Verification items for the finished model (mm, model axes). A direction names the side the tool comes from. Round coordinates to 2 decimals unless told otherwise and drop trailing zeros. Order: outer loops, then holes, each group sorted by start corner. A loop starts at its lowest first (then second) coordinate and runs counter-clockwise, first axis right, second up. Notation, with made-up numbers: (-11, 28.5) -> (46, 28.5) arc R29 ccw to (46, 63.5) -> close; hole circle Ø8 at (76.25, -10). An arc over 180 degrees is marked (long way). Return JSON: item names as keys, results as strings. Group by question number.
1) Section check B-B on y = -21. Enter the section's corners in (x, z).
2) Section check A-A on x = 363. Enter the section's corners in (y, z), plus the area to 3 significant figures.
3) Depth check by flat-ended pin: pin 1 (8 mm diameter, centred on x = 1498.6, z = -27.305, fed in from -Y); pin 2 (5.5 mm diameter, centred on x = 3.81, z = -33.34, fed in from +Y); pin 3 (8 mm diameter, centred on x = 532.5, y = -24, fed in from -Z); pin 4 (6 mm diameter, centred on y = -29.5, z = -4.5, fed in from -X). Enter the tip coordinate at first touch or a pass-through.
4) Tool access check on faces 1 (the flat face through (742, 0, -28)), 2 (the flat face through (742, -2.591, -28)). Record the directions out of +Z, -Z, +X, -X, +Y, -Y that give a thin tool (end or side, any length) a straight path to the whole face; none if there is none.
5) Scan lines: L1, parallel to Z at x = 1498.6, y = -0.85; L2, parallel to Z at x = 3.81, y = -0.65; L3, parallel to Y at x = 86.5, z = -31. Record each from-to range of solid material in increasing order.
```python
from build123d import *

# Parameters (mm, degrees)
BASE_FLANGE1_DEPTH               = 2.5908
EDGE_FLANGE1_STRIP_W             = 15.4432
EDGE_FLANGE1_STRIP_H             = 2.5908
EDGE_FLANGE1_STRIP_CUT_DEPTH     = 1524
EDGE_FLANGE1_DEPTH               = 1524
F_17_64_0_26563_DIAMETER_HOLE1_D = 6.747002
FILLET1_R                        = 3.175
F_17_64_0_26563_DIAMETER_HOLE2_D = 6.747002


# Sheet-metal steps are written as plain solids
with BuildPart() as part:
    # Sketch2 → Base-Flange1 (new body)
    with BuildSketch(Plane(origin=(0, 0, 0), x_dir=(1, 0, 0), z_dir=(0, 1, 0))):
        Polygon((0, 0), (1524, 0), (1524, 50.8), (-19.05, 50.8), (-19.05, 19.05), (0, 9.525), align=None)
    extrude(amount=-BASE_FLANGE1_DEPTH)

    # Edge-Flange1 strip (across the edge) → Edge-Flange1 strip cut (cut)
    with BuildSketch(Plane(origin=(1524, -2.5908, 0), x_dir=(0, 0, -1), z_dir=(-1, 0, 0))):
        with Locations((-2.5908, -1.2954)):
            Rectangle(EDGE_FLANGE1_STRIP_W, EDGE_FLANGE1_STRIP_H)
    extrude(amount=EDGE_FLANGE1_STRIP_CUT_DEPTH, mode=Mode.SUBTRACT)

    # Edge-Flange1 section (across the edge) → Edge-Flange1 (add)
    with BuildSketch(Plane(origin=(1524, -2.5908, 0), x_dir=(0, 0, -1), z_dir=(-1, 0, 0))):
        with BuildLine():
            Line((0, 2.54), (0, 48.2092))
            Line((0, 48.2092), (2.5908, 48.2092))
            Line((2.5908, 48.2092), (2.5908, 2.54))
            ThreePointArc((2.5908, 2.54), (3.334748776, 0.743948776), (5.1308, 0))
            Line((5.1308, 0), (5.1308, -2.5908))
            ThreePointArc((5.1308, -2.5908), (1.502776527, -1.088023473), (0, 2.54))
        make_face()
    extrude(amount=EDGE_FLANGE1_DEPTH)

    # 17/64 (0.26563) Diameter Hole1 (through all)
    with Locations(Plane(origin=(0, 0, 0), x_dir=(1, 0, 0), z_dir=(0, 1, 0))):
        with Locations((1498.6, 27.305)):
            Hole(F_17_64_0_26563_DIAMETER_HOLE1_D / 2)

    # Fillet1
    fillet1_edges = [part.edges().sort_by_distance(p)[0] for p in [
        (0, -1.2954, -9.525),
        (-19.05, -1.2954, -19.05),
        (-19.05, -1.2954, -50.8),
        (1524, -1.2954, -50.8),
        (1524, -50.8, -1.2954),
        (0, -50.8, -1.2954),
    ]]
    fillet(fillet1_edges, radius=FILLET1_R)

    # 17/64 (0.26563) Diameter Hole2 (through all)
    with Locations(Plane(origin=(0, 0, 0), x_dir=(1, 0, 0), z_dir=(0, 1, 0))):
        with Locations((3.81, 33.3375)):
            Hole(F_17_64_0_26563_DIAMETER_HOLE2_D / 2)


solid = part.part
```
Check result:
{
 "1": {"outline": "(0, -2.59) -> (1524, -2.59) -> (1524, 0) -> (0, 0) -> close"},
 "2": {"outline": "(-50.8, -2.59) -> (-5.13, -2.59) arc R2.54 cw to (-2.59, -5.13) -> (-2.59, -50.8) -> (0, -50.8) -> (0, -5.13) arc R5.13 ccw to (-5.13, 0) -> (-50.8, 0) -> close", "area": "252 mm^2"},
 "3": {"pin 1": "y = -2.59", "pin 2": "through", "pin 3": "z = -2.59", "pin 4": "x = 0"},
 "4": {"face 1": "+Z, -Z, +X, -X, +Y", "face 2": "-Z, +X, -X, -Y"},
 "5": {"L1": "-50.8 to -30.68, -23.93 to -2.3", "L2": "-50.8 to -36.71, -29.96 to -2.63", "L3": "-2.59 to 0"}
}
